```python
from build123d import *

# Parameters (mm, degrees)
F2_R          = 6.482371
F3_DEPTH      = 32.004
F3_DEPTH_BACK = 32.004


with BuildPart() as f1:
    # F0 (on Front) → F1 (revolve)
    with BuildSketch(Plane.XZ):
        Polygon((6.721209, 55.426951), (0, 55.426951), (0, 27.805546), (0, 25.227549), (0, 0), (0, -21.728838), (0, -29.483447), (10.483314, -29.483447), (10.483314, -14.915559), (6.721209, -14.915559), (6.721209, 25.227549), (4.879782, 25.227549), (4.879782, 27.805546), (6.721209, 27.805546), (6.721209, 42.352822), (6.721209, 48.06124), align=None)
    revolve(axis=Axis((0, 0, 27.713476), (0, 0, 1)))

    # F2 (on Front) → F3 (join, two sides)
    with BuildSketch(Plane.XZ) as f3_sk:
        with Locations((0, 42.905249)):
            Circle(F2_R)
    extrude(amount=F3_DEPTH)
    extrude(f3_sk.sketch, amount=-F3_DEPTH_BACK)


solid = f1.part
```
Design review of the part built by this model. Coordinates are the model's own, in mm. A direction names the side the tool comes from. Coordinates: 2 decimals unless noted, no trailing zeros. Loops run counter-clockwise (first coordinate to the right, second up) from the corner with the lowest first, then second, coordinate; pieces in that order, holes last. Notation, with made-up numbers: (85.5, 88.25) -> (97.5, 88.25) arc R10 cw to (97.5, 102.25) -> close; hole circle Ø5 at (-19, 31). An arc over 180 degrees is marked (long way). Answer as a JSON object with one key per item and string values.
Q1. Clearance check with flat-ended pins moving along their axes: pin 1 Ø4 at (y, z) = (3, 34.5) entering from +X; pin 2 Ø1 at (x, y) = (1, 8.5) entering from +Z; pin 3 Ø2 at (y, z) = (-4, -10) entering from -X. State where each tip first meets the part, or that it passes through.
Answer block:
{"pin 1": "stops at x = 6.65", "pin 2": "stops at z = 49.37", "pin 3": "stops at x = -6.01"}
Q2. The part is to be moulded in two halves that separate along Z. For faces 5 (the flat face through (0, 0, -29.483)), 6 (the flat face through (0, 0, 55.427)), 7 (the cylindrical face through (10, 3.15, -22.1)), 8 (the cylindrical face through (4.654, 1.466, 26.535)), say which applies: +Z half, -Z half, draft (parallel to the pull), parting line (faces both ways), or undercut.
Answer block:
{"face 5": "-Z half", "face 6": "+Z half", "face 7": "draft", "face 8": "undercut"}
Q3. Take a section at D-D on y = 8.5. Give the boundary of the cut face in (x, z), plus the area to 3 significant figures.
Answer block:
{"outline": "circle Ø12.96 at (0, 42.91); (-6.14, -29.48) -> (6.14, -29.48) -> (6.14, -14.92) -> (-6.14, -14.92) -> close", "area": "311 mm^2"}
Q4. Take a section at B-B on y = 0. Give the boundary of the cut face in (x, z).
Answer block:
{"outline": "(-10.48, -29.48) -> (10.48, -29.48) -> (10.48, -14.92) -> (6.72, -14.92) -> (6.72, 25.23) -> (4.88, 25.23) -> (4.88, 27.81) -> (6.72, 27.81) -> (6.72, 55.43) -> (-6.72, 55.43) -> (-6.72, 27.81) -> (-4.88, 27.81) -> (-4.88, 25.23) -> (-6.72, 25.23) -> (-6.72, -14.92) -> (-10.48, -14.92) -> close"}
Q5. Tool access review of faces 1 (the cylindrical face through (2.991, -16.678, 37.154)), 2 (the flat face through (0, 32.004, 43)), 3 (the cylindrical face through (2.991, 16.678, 37.154)), 4 (the flat face through (4, 4, 27.806)): name each direction out of +Z, -Z, +X, -X, +Y, -Y from which nothing blocks a thin tool from reaching the whole face with its end or side.
Answer block:
{"face 1": "-Y", "face 2": "+Z, -Z, +X, -X, +Y", "face 3": "+Y", "face 4": "none"}
Q6. Take a section at C-C on z = 10. Give the boundary of the cut face in (x, y).
Answer block:
{"outline": "circle Ø13.44 at (0, 0)"}
Q7. Take a section at A-A on x = 0. Give the boundary of the cut face in (y, z).
Answer block:
{"outline": "(-32, 36.42) -> (-6.72, 36.42) -> (-6.72, 27.81) -> (-4.88, 27.81) -> (-4.88, 25.23) -> (-6.72, 25.23) -> (-6.72, -14.92) -> (-10.48, -14.92) -> (-10.48, -29.48) -> (10.48, -29.48) -> (10.48, -14.92) -> (6.72, -14.92) -> (6.72, 25.23) -> (4.88, 25.23) -> (4.88, 27.81) -> (6.72, 27.81) -> (6.72, 36.42) -> (32, 36.42) -> (32, 49.39) -> (6.72, 49.39) -> (6.72, 55.43) -> (-6.72, 55.43) -> (-6.72, 49.39) -> (-32, 49.39) -> close"}
Q8. To check wall thickness, follow L1, parallel to Z at x = 3, y = -5; L2, parallel to Y at x = -1.5, z = 18.5; L3, parallel to Z at x = -3.5, y = 23. State the ranges of each line that lie inside material, in increasing order.
Answer block:
{"L1": "z = -29.48 to 25.23, 27.81 to 55.43", "L2": "y = -6.55 to 6.55", "L3": "z = 37.45 to 48.36"}
